from build123d import *

# Parameters (mm, degrees)
SKETCH1_R           = 1.55
BOSS_EXTRUDE1_DEPTH = 5
SKETCH2_W           = 98
SKETCH2_H           = 8
BOSS_EXTRUDE2_DEPTH = 55
BOSS_EXTRUDE3_DEPTH = 15
FILLET2_R           = 5
CUT_EXTRUDE1_DEPTH  = 15
FILLET3_R           = 1


with BuildPart() as part:
    # Sketch1 → Boss-Extrude1 (new body)
    with BuildSketch(Plane.XY):
        with BuildLine():
            Line((-49, 0), (-49, -100))
            Line((-49, -100), (49, -100))
            Line((49, -100), (49, 0))
            ThreePointArc((49, 0), (44.625, 4.375), (40.25, 0))
            ThreePointArc((40.25, 0), (0, -40.25), (-40.25, 0))
            ThreePointArc((-40.25, 0), (-44.625, 4.375), (-49, 0))
        make_face()
        with Locations((0, -44.5)):
            Circle(SKETCH1_R, mode=Mode.SUBTRACT)
        with Locations((-31.466251763, -31.466251763)):
            Circle(SKETCH1_R, mode=Mode.SUBTRACT)
        with Locations((-44.5, 0)):
            Circle(SKETCH1_R, mode=Mode.SUBTRACT)
        with Locations((44.5, 0)):
            Circle(SKETCH1_R, mode=Mode.SUBTRACT)
        with Locations((31.466251763, -31.466251763)):
            Circle(SKETCH1_R, mode=Mode.SUBTRACT)
        with BuildLine():
            Line((-12.5, -92), (-29, -92))
            ThreePointArc((-29, -92), (-32.535533906, -90.535533906), (-34, -87))
            Line((-34, -87), (-34, -43.878620458))
            Line((-34, -43.878620458), (-10, -57.735026919))
            ThreePointArc((-10, -57.735026919), (-8.169872981, -59.565153938), (-7.5, -62.065153938))
            Line((-7.5, -62.065153938), (-7.5, -87))
            ThreePointArc((-7.5, -87), (-8.964466094, -90.535533906), (-12.5, -92))
        make_face(mode=Mode.SUBTRACT)
        with BuildLine():
            Line((10, -57.735026919), (34, -43.878620458))
            Line((34, -43.878620458), (34, -87))
            ThreePointArc((34, -87), (32.535533906, -90.535533906), (29, -92))
            Line((29, -92), (12.5, -92))
            ThreePointArc((12.5, -92), (8.964466094, -90.535533906), (7.5, -87))
            Line((7.5, -87), (7.5, -62.065153938))
            ThreePointArc((7.5, -62.065153938), (8.169872981, -59.565153938), (10, -57.735026919))
        make_face(mode=Mode.SUBTRACT)
    extrude(amount=BOSS_EXTRUDE1_DEPTH)

    # Sketch2 → Boss-Extrude2 (add)
    with BuildSketch(Plane.XY.offset(5)):
        with Locations((0, -96)):
            Rectangle(SKETCH2_W, SKETCH2_H)
    extrude(amount=BOSS_EXTRUDE2_DEPTH)

    # Sketch3 → Boss-Extrude3 (add)
    with BuildSketch(Plane(origin=(49, 0, 0), x_dir=(0, 0, -1), z_dir=(1, 0, 0))):
        Polygon((-5, -35), (-32.5, -92), (-5, -92), align=None)
    boss_extrude3 = extrude(amount=-BOSS_EXTRUDE3_DEPTH)

    # Mirror1: Boss-Extrude3 across plane
    add(boss_extrude3.mirror(Plane(origin=(0, 0, 0), x_dir=(0, 0, 1), z_dir=(1, 0, 0))))

    # Fillet2
    fillet2_edges = [part.edges().sort_by_distance(p)[0] for p in [
        (41.5, -92, 32.5),
        (-41.5, -92, 32.5),
        (-34, -43.878620458, 2.5),
        (34, -43.878620458, 2.5),
        (-49, -96, 60),
        (49, -96, 60),
    ]]
    fillet(fillet2_edges, radius=FILLET2_R)

    # Sketch4 → Cut-Extrude1 (cut)
    with BuildSketch(Plane(origin=(0, -92, 0), x_dir=(1, 0, 0), z_dir=(0, 1, 0))):
        with BuildLine():
            Line((-17.6, -45), (-17.6, -15))
            ThreePointArc((-17.6, -15), (-15, -12.4), (-12.4, -15))
            Line((-12.4, -15), (-12.4, -45))
            ThreePointArc((-12.4, -45), (-15, -47.6), (-17.6, -45))
        make_face()
        with BuildLine():
            Line((17.6, -45), (17.6, -15))
            ThreePointArc((17.6, -15), (15, -12.4), (12.4, -15))
            Line((12.4, -15), (12.4, -45))
            ThreePointArc((12.4, -45), (15, -47.6), (17.6, -45))
        make_face()
    extrude(amount=-CUT_EXTRUDE1_DEPTH, mode=Mode.SUBTRACT)

    # Fillet3
    # the kernel refuses this fillet: 1 mm, written as the material it takes off along each edge
    with BuildSketch(Plane(origin=(49, -106, 0), x_dir=(-1, 0, 0), z_dir=(0, 1, 0))) as fillet3_piece_1:
        with BuildLine():
            CenterArc((FILLET3_R, FILLET3_R), FILLET3_R, 180, 90)
            Line((0, FILLET3_R), (-FILLET3_R * 0.02, FILLET3_R))
            Line((-FILLET3_R * 0.02, FILLET3_R), (-FILLET3_R * 0.02, -FILLET3_R * 0.02))
            Line((-FILLET3_R * 0.02, -FILLET3_R * 0.02), (FILLET3_R, -FILLET3_R * 0.02))
            Line((FILLET3_R, -FILLET3_R * 0.02), (FILLET3_R, 0))
        make_face()
    extrude(amount=112, mode=Mode.SUBTRACT)
    with BuildSketch(Plane(origin=(-49, 6, 0), x_dir=(0, 0, 1), z_dir=(0, -1, 0))) as fillet3_piece_2:
        with BuildLine():
            CenterArc((FILLET3_R, -FILLET3_R), FILLET3_R, 90, 90)
            Line((0, -FILLET3_R), (-FILLET3_R * 0.02, -FILLET3_R))
            Line((-FILLET3_R * 0.02, -FILLET3_R), (-FILLET3_R * 0.02, FILLET3_R * 0.02))
            Line((-FILLET3_R * 0.02, FILLET3_R * 0.02), (FILLET3_R, FILLET3_R * 0.02))
            Line((FILLET3_R, FILLET3_R * 0.02), (FILLET3_R, 0))
        make_face()
    extrude(amount=112, mode=Mode.SUBTRACT)


solid = part.part
The listing builds one solid part. Answer for the finished solid, in the listing's coordinates (mm). A direction names the side the tool comes from. Give positions to 0.01 mm unless a question says otherwise; leave off trailing zeros. Order: outer loops, then holes, each group sorted by start corner. A loop starts at its lowest first (then second) coordinate and runs counter-clockwise, first axis right, second up. Notation, with made-up numbers: (88, -10) - (144, -10) arc R19 ccw to (144, 27) - close; hole circle Ø6 at (36, 21.25). An arc over 180 degrees is marked (long way). Answer as CSV lines item,"result".
Q1. A cutting plane is placed at C-C, the plane y = -19. Determine the outline of the cut face in (x, z).
Answer key:
outline,"(-49, 1) arc R1 ccw to (-48, 0) - (-35.48, 0) - (-35.48, 5) - (-49, 5) - close; (35.48, 0) - (48, 0) arc R1 ccw to (49, 1) - (49, 5) - (35.48, 5) - close"
Q2. A cutting plane is placed at B-B, the plane z = 28.5. Determine the outline of the cut face in (x, y).
Answer key:
outline,"(-49, -100) - (-17.6, -100) - (-17.6, -92) - (-34, -92) - (-34, -83.71) - (-49, -83.71) - close; (-12.4, -100) - (12.4, -100) - (12.4, -92) - (-12.4, -92) - close; (17.6, -100) - (49, -100) - (49, -83.71) - (34, -83.71) - (34, -92) - (17.6, -92) - close"
Q3. Determine the mould class of faces 1 (the face through (-30.034, -32.06, 2.465)), 2 (the face through (-33, -91, 5)), 3 (the face through (-15.1, -95.9, 12.4)) for opening direction Z: pulls with the +Z half, pulls with the -Z half, needs draft (parallel to the pull), parting line crosses it, or undercut.
Answer key:
face 1,"needs draft"
face 2,"pulls with the +Z half"
face 3,"undercut"
Q4. Each of these flat-tipped pins is pushed along its axis until it touches: pin 1 Ø3 at (x, y) = (-44.5, 0) entering from -Z; pin 2 Ø3.5 at (x, y) = (0, -44.5) entering from -Z; pin 3 Ø18 at (x, z) = (-7.5, 38.5) entering from +Y; pin 4 Ø2.5 at (x, y) = (32.5, -88.5) entering from +Z. Where does it stop, or does it pass through?
Answer key:
pin 1,"passes through"
pin 2,"stops at z = 0"
pin 3,"stops at y = -92"
pin 4,"stops at z = 5"
Q5. A cutting plane is placed at A-A, the plane x = 0. Determine the outline of the cut face in (y, z).
Answer key:
outline,"(-100, 0) - (-46.05, 0) - (-46.05, 5) - (-92, 5) - (-92, 60) - (-100, 60) - close; (-42.95, 0) - (-40.25, 0) - (-40.25, 5) - (-42.95, 5) - close"
Q6. Straight lines are drawn through the part: L1, parallel to X at y = -78, z = 16; L2, parallel to Y at x = 44.5, z = 3; L3, parallel to Y at x = 25, z = 20. For each, find the intervals that lie inside material, in ascending order.
Answer key:
L1,"x = -49 to -34, 34 to 49"
L2,"y = -100 to -1.55, 1.55 to 4.37"
L3,"y = -100 to -92"
Q7. Which of the six approach directions +Z, -Z, +X, -X, +Y, -Y give full straight-line access (tool end or side, diameter ignored) to faces 4 (the face through (-41.605, -61.707, 17.885)), 5 (the face through (-4, -44, 5)), 6 (the face through (7.5, -75, 2)), 7 (the face through (17.6, -96, 30))?
Answer key:
face 4,"+Z, +X, -X, +Y"
face 5,"+Z, +Y"
face 6,"+Z, -Z"
face 7,"+Y, -Y"
Q8. A cutting plane is placed at D-D, the plane x = -16. Determine the outline of the cut face in (y, z), and give its area (3 significant figures).
Answer key:
outline,"(-100, 0) - (-92, 0) - (-92, 12.6) - (-100, 12.6) - close; (-100, 47.4) - (-92, 47.4) - (-92, 60) - (-100, 60) - close; (-54.27, 0) - (-36.93, 0) - (-36.93, 5) - (-54.27, 5) - close"
area,"288 mm^2"
